from build123d import *

# Parameters (mm, degrees)
BOSS_EXTRUDE1_DEPTH = 10
CUT_EXTRUDE1_REACH  = 12
SKETCH3_R           = 5
CUT_EXTRUDE3_REACH  = 12
SKETCH2_R           = 5


with BuildPart() as part:
    # Sketch1 → Boss-Extrude1 (new body)
    with BuildSketch(Plane(origin=(0, 0, 0), x_dir=(0, 0, -1), z_dir=(1, 0, 0))):
        with BuildLine():
            Line((-110, 15), (110, 15))
            ThreePointArc((110, 15), (125, 0), (110, -15))
            Line((110, -15), (-110, -15))
            ThreePointArc((-110, -15), (-125, 0), (-110, 15))
        make_face()
    extrude(amount=BOSS_EXTRUDE1_DEPTH)

    # Sketch3 → Cut-Extrude1 (cut, up to next)
    with BuildSketch(Plane.ZY, mode=Mode.PRIVATE) as cut_extrude1_sk1:
        with Locations((110, 0)):
            Circle(SKETCH3_R)
    cut_extrude1_tool1 = extrude(cut_extrude1_sk1.sketch, amount=-CUT_EXTRUDE1_REACH, mode=Mode.PRIVATE) & part.part
    add(cut_extrude1_tool1.solids().sort_by_distance((0, 0, 110))[0], mode=Mode.SUBTRACT)

    # Sketch2 → Cut-Extrude3 (cut, up to next)
    with BuildSketch(Plane.ZY, mode=Mode.PRIVATE) as cut_extrude3_sk1:
        with Locations((-110, 0)):
            Circle(SKETCH2_R)
    cut_extrude3_tool1 = extrude(cut_extrude3_sk1.sketch, amount=-CUT_EXTRUDE3_REACH, mode=Mode.PRIVATE) & part.part
    add(cut_extrude3_tool1.solids().sort_by_distance((0, 0, -110))[0], mode=Mode.SUBTRACT)


solid = part.part
The model under review builds one solid part; all positions refer to its coordinate system, in mm. Give positions to 0.01 mm unless a question says otherwise; leave off trailing zeros. Order: outer loops, then holes, each group sorted by start corner. A loop starts at its lowest first (then second) coordinate and runs counter-clockwise, first axis right, second up. Notation, with made-up numbers: (88, 8) -> (104, 8) arc R12 cw to (104, 25) -> close; hole circle Ø1 at (-6, -15.75). An arc over 180 degrees is marked (long way). Write item = value, one per line. Start each with the question number.
(1) For L1, parallel to Y at x = 5.75, z = 110; L2, parallel to Z at x = 4.25, y = 3; L3, parallel to Z at x = 6.5, y = 5.5, list the stretches that pass through material, from the lowest coordinate up. Write a range as from..to.
(2) Take a section at B-B (x = 6.75). Write out the cut boundary in (y, z), plus the area to 3 significant figures.
(3) Take a section at A-A (y = 0). Write out the cut boundary in (x, z), plus the area to 3 significant figures.
(4) Draft analysis for pull direction Y (two halves, no side actions). For faces 1 (the flat face through (10, 0, -2)), 2 (the cylindrical face through (5, 0, -125)), 3 (the cylindrical face through (4.93, -1.915, -105.381)), state which applies: +Y half, -Y half, draft (parallel to the pull), parting line (faces both ways), or undercut.
(5) Take a section at C-C (y = 10). Write out the cut boundary in (x, z), plus the area to 3 significant figures.
(6) For pin 1 Ø1 at (x, y) = (5, 9.5) entering from -Z; pin 2 Ø1.5 at (x, y) = (2.5, 10) entering from +Z, all flat-tipped, find the tip position at first contact; note any pin that passes through.
Returned:
q1.L1 = -15..-5, 5..15
q1.L2 = -124.7..-114, -106..106, 114..124.7
q1.L3 = -123.96..123.96
q2.outline = (-15, -110) arc R15 ccw to (15, -110) -> (15, 110) arc R15 ccw to (-15, 110) -> close; hole circle Ø10 at (0, -110); hole circle Ø10 at (0, 110)
q2.area = 7,150 mm²
q3.outline = (0, -125) -> (10, -125) -> (10, -115) -> (0, -115) -> close; (0, -105) -> (10, -105) -> (10, 105) -> (0, 105) -> close; (0, 115) -> (10, 115) -> (10, 125) -> (0, 125) -> close
q3.area = 2,300 mm²
q4.face_1 = draft
q4.face_2 = parting line
q4.face_3 = undercut
q5.outline = (0, -121.18) -> (10, -121.18) -> (10, 121.18) -> (0, 121.18) -> close
q5.area = 2,420 mm²
q6.pin_1 = -122
q6.pin_2 = 121.81
